from build123d import *

# Parameters (mm, degrees)
F0_R         = 16.5
F0_R_2       = 3.5170103203
F1_DEPTH     = 40
F2_R         = 16.5
F3_DEPTH     = 38
F4_W         = 50
F4_H         = 34
F5_DEPTH     = 4.5
F6_W         = 50
F6_H         = 2.5
F7_DEPTH     = 4.5
F8_T1_DEPTH  = 1.5
F8_T3_DEPTH  = 24
F8_T5_DEPTH  = 32.3129968036
F8_T7_DEPTH  = 12.8102496977
F8_T9_DEPTH  = 43
F8_T11_DEPTH = 26.1042093904
F8_T13_DEPTH = 10
F8_T20_ANGLE = 69.5823366889
F8_T22_ANGLE = 20.4176633111
F8_T24_ANGLE = 90
F8_T26_ANGLE = 90
F8_T28_ANGLE = 90
F8_T30_ANGLE = 90
F8_T32_ANGLE = 90
F9_R         = 1


# Not quite as in the source:
# - a fillet or chamfer that OpenCascade refuses, or shapes differently, is made with other operations: its cross-section is extruded or revolved along the edge and cut away or added


with BuildPart() as f1:
    # F0 (on Top) → F1 (new body)
    with BuildSketch(Plane.XY):
        with BuildLine():
            Line((0, 38), (0, 0))
            Line((0, 0), (12.5, 0))
            Line((12.5, 0), (12.5, -4.5))
            Line((12.5, -4.5), (62.5, -4.5))
            Line((62.5, -4.5), (62.5, 0))
            Line((62.5, 0), (75, 0))
            Line((75, 0), (75, 21.1042093904))
            ThreePointArc((75, 21.1042093904), (71.4247434001, 32.5159491456), (61.9772195759, 39.8476991132))
            Line((61.9772195759, 39.8476991132), (31.6943034009, 51.120442806))
            ThreePointArc((31.6943034009, 51.120442806), (29.2915599077, 51.7783562025), (26.8102496977, 52))
            Line((26.8102496977, 52), (14, 52))
            ThreePointArc((14, 52), (4.1005050634, 47.8994949366), (0, 38))
        make_face()
        with Locations((54.5, 20.5)):
            Circle(F0_R, mode=Mode.SUBTRACT)
        with BuildLine():
            ThreePointArc((4, 38), (6.9289321881, 45.0710678119), (14, 48))
            Line((14, 48), (24, 48))
            ThreePointArc((24, 48), (31.0710678119, 45.0710678119), (34, 38))
            Line((34, 38), (34, 14))
            ThreePointArc((34, 14), (31.0710678119, 6.9289321881), (24, 4))
            Line((24, 4), (14, 4))
            ThreePointArc((14, 4), (6.9289321881, 6.9289321881), (4, 14))
            Line((4, 14), (4, 38))
        make_face(mode=Mode.SUBTRACT)
        with Locations((41.3257834749, 40.5812550323)):
            Circle(F0_R_2, mode=Mode.SUBTRACT)
        with Locations((54.5, 20.5)):
            Circle(F0_R)
    extrude(amount=F1_DEPTH)

    # F2 (on face) → F3 (cut)
    with BuildSketch(Plane.XY.offset(40)):
        with Locations((54.5, 20.5)):
            Circle(F2_R)
    extrude(amount=-F3_DEPTH, mode=Mode.SUBTRACT)

    # F4 (on face) → F5 (cut)
    with BuildSketch(Plane.XZ.offset(4.5)):
        with Locations((37.5, 17)):
            Rectangle(F4_W, F4_H)
    extrude(amount=-F5_DEPTH, mode=Mode.SUBTRACT)

    # F6 (on face) → F7 (cut)
    with BuildSketch(Plane(origin=(0, 0, 34), x_dir=(1, 0, 0), z_dir=(0, 0, -1))):
        with Locations((37.5, 1.25)):
            Rectangle(F6_W, F6_H)
    extrude(amount=-F7_DEPTH, mode=Mode.SUBTRACT)

    # F8: fillet of radius 2 on 6 edges, made by hand

    # F8_s2 → F8_t1 (join)
    with BuildSketch(Plane.XY.offset(38.5)):
        with BuildLine():
            ThreePointArc((10.5, 0), (11.9142135624, -0.5857864376), (12.5, -2))
            Line((12.5, -2), (12.5, 0))
            Line((12.5, 0), (10.5, 0))
        make_face()
        with BuildLine():
            ThreePointArc((64.5, 0), (63.0857864376, -0.5857864376), (62.5, -2))
            Line((62.5, -2), (62.5, 0))
            Line((62.5, 0), (64.5, 0))
        make_face()
    extrude(amount=F8_T1_DEPTH)

    # F8_s4 → F8_t3 (cut)
    with BuildSketch(Plane.XZ.offset(-38)):
        with BuildLine():
            ThreePointArc((36, 40), (34.5857864376, 39.4142135624), (34, 38))
            Line((34, 38), (34, 40))
            Line((34, 40), (36, 40))
        make_face()
        with BuildLine():
            ThreePointArc((2, 40), (3.4142135624, 39.4142135624), (4, 38))
            Line((4, 38), (4, 40))
            Line((4, 40), (2, 40))
        make_face()
    extrude(amount=F8_T3_DEPTH, mode=Mode.SUBTRACT)

    # F8_s6 → F8_t5 (cut)
    with BuildSketch(Plane(origin=(41.4063945876, -15.4134321387, 0), x_dir=(0, 0, 1), z_dir=(-0.9371744861, 0.3488609788, 0))):
        with BuildLine():
            ThreePointArc((40, 56.9656804247), (39.4142135624, 58.3798939871), (38, 58.9656804247))
            Line((38, 58.9656804247), (40, 58.9656804247))
            Line((40, 58.9656804247), (40, 56.9656804247))
        make_face()
    extrude(amount=F8_T5_DEPTH, mode=Mode.SUBTRACT)

    # F8_s8 → F8_t7 (cut)
    with BuildSketch(Plane.YZ.offset(14)):
        with BuildLine():
            ThreePointArc((50, 40), (51.4142135624, 39.4142135624), (52, 38))
            Line((52, 38), (52, 40))
            Line((52, 40), (50, 40))
        make_face()
    extrude(amount=F8_T7_DEPTH, mode=Mode.SUBTRACT)

    # F8_s10 → F8_t9 (cut)
    with BuildSketch(Plane.XZ.offset(-38)):
        with BuildLine():
            ThreePointArc((2, 40), (0.5857864376, 39.4142135624), (0, 38))
            Line((0, 38), (0, 40))
            Line((0, 40), (2, 40))
        make_face()
    extrude(amount=F8_T9_DEPTH, mode=Mode.SUBTRACT)

    # F8_s12 → F8_t11 (cut)
    with BuildSketch(Plane.XZ.offset(-21.1042093904)):
        with BuildLine():
            ThreePointArc((73, 40), (74.4142135624, 39.4142135624), (75, 38))
            Line((75, 38), (75, 40))
            Line((75, 40), (73, 40))
        make_face()
    extrude(amount=F8_T11_DEPTH, mode=Mode.SUBTRACT)

    # F8_s14 → F8_t13 (cut)
    with BuildSketch(Plane.YZ.offset(14)):
        with BuildLine():
            ThreePointArc((2, 40), (3.4142135624, 39.4142135624), (4, 38))
            Line((4, 38), (4, 40))
            Line((4, 40), (2, 40))
        make_face()
        with BuildLine():
            ThreePointArc((50, 40), (48.5857864376, 39.4142135624), (48, 38))
            Line((48, 38), (48, 40))
            Line((48, 40), (50, 40))
        make_face()
    extrude(amount=F8_T13_DEPTH, mode=Mode.SUBTRACT)

    # F8_s15 → F8_t16 (revolve, cut)
    with BuildSketch(Plane.XZ.offset(-20.5)):
        with BuildLine():
            ThreePointArc((73, 40), (71.5857864376, 39.4142135624), (71, 38))
            Line((71, 38), (71, 40))
            Line((71, 40), (73, 40))
        make_face()
    revolve(axis=Axis((54.5, 20.5, 40), (0, 0, 1)), mode=Mode.SUBTRACT)

    # F8_s17 → F8_t18 (revolve, cut)
    with BuildSketch(Plane.XZ.offset(-40.5812550323)):
        with BuildLine():
            ThreePointArc((46.8427937951, 40), (45.4285802328, 39.4142135624), (44.8427937951, 38))
            Line((44.8427937951, 38), (44.8427937951, 40))
            Line((44.8427937951, 40), (46.8427937951, 40))
        make_face()
    revolve(axis=Axis((41.3257834749, 40.5812550323, 40), (0, 0, 1)), mode=Mode.SUBTRACT)

    # F8_s19 → F8_t20 (revolve, cut)
    with BuildSketch(Plane.XZ.offset(-21.1042093904)):
        with BuildLine():
            ThreePointArc((73, 40), (74.4142135624, 39.4142135624), (75, 38))
            Line((75, 38), (75, 40))
            Line((75, 40), (73, 40))
        make_face()
    revolve(axis=Axis((55, 21.1042093904, 40), (0, 0, 1)), revolution_arc=F8_T20_ANGLE, mode=Mode.SUBTRACT)

    # F8_s21 → F8_t22 (revolve, cut)
    with BuildSketch(Plane(origin=(11.1234784125, -4.140688446, 0), x_dir=(0, 0, 1), z_dir=(0.9371744861, -0.3488609788, 0))):
        with BuildLine():
            ThreePointArc((38, -58.9656804247), (39.4142135624, -58.3798939871), (40, -56.9656804247))
            Line((40, -56.9656804247), (40, -58.9656804247))
            Line((40, -58.9656804247), (38, -58.9656804247))
        make_face()
    revolve(axis=Axis((26.8102496977, 38, 40), (0, 0, 1)), revolution_arc=F8_T22_ANGLE, mode=Mode.SUBTRACT)

    # F8_s23 → F8_t24 (revolve, cut)
    with BuildSketch(Plane.YZ.offset(14)):
        with BuildLine():
            ThreePointArc((50, 40), (51.4142135624, 39.4142135624), (52, 38))
            Line((52, 38), (52, 40))
            Line((52, 40), (50, 40))
        make_face()
    revolve(axis=Axis((14, 38, 40), (0, 0, 1)), revolution_arc=F8_T24_ANGLE, mode=Mode.SUBTRACT)

    # F8_s25 → F8_t26 (revolve, cut)
    with BuildSketch(Plane.YZ.offset(24)):
        with BuildLine():
            ThreePointArc((50, 40), (48.5857864376, 39.4142135624), (48, 38))
            Line((48, 38), (48, 40))
            Line((48, 40), (50, 40))
        make_face()
    revolve(axis=Axis((24, 38, 40), (0, 0, -1)), revolution_arc=F8_T26_ANGLE, mode=Mode.SUBTRACT)

    # F8_s27 → F8_t28 (revolve, cut)
    with BuildSketch(Plane.XZ.offset(-14)):
        with BuildLine():
            ThreePointArc((36, 40), (34.5857864376, 39.4142135624), (34, 38))
            Line((34, 38), (34, 40))
            Line((34, 40), (36, 40))
        make_face()
    revolve(axis=Axis((24, 14, 40), (0, 0, -1)), revolution_arc=F8_T28_ANGLE, mode=Mode.SUBTRACT)

    # F8_s29 → F8_t30 (revolve, cut)
    with BuildSketch(Plane.YZ.offset(14)):
        with BuildLine():
            ThreePointArc((2, 40), (3.4142135624, 39.4142135624), (4, 38))
            Line((4, 38), (4, 40))
            Line((4, 40), (2, 40))
        make_face()
    revolve(axis=Axis((14, 14, 40), (0, 0, -1)), revolution_arc=F8_T30_ANGLE, mode=Mode.SUBTRACT)

    # F8_s31 → F8_t32 (revolve, cut)
    with BuildSketch(Plane.XZ.offset(-38)):
        with BuildLine():
            ThreePointArc((2, 40), (3.4142135624, 39.4142135624), (4, 38))
            Line((4, 38), (4, 40))
            Line((4, 40), (2, 40))
        make_face()
    revolve(axis=Axis((14, 38, 40), (0, 0, -1)), revolution_arc=F8_T32_ANGLE, mode=Mode.SUBTRACT)

    # F9
    f9_edges = [f1.edges().sort_by_distance(p)[0] for p in [
        (37.5, -4.5, 40),
    ]]
    fillet(f9_edges, radius=F9_R)


solid = f1.part
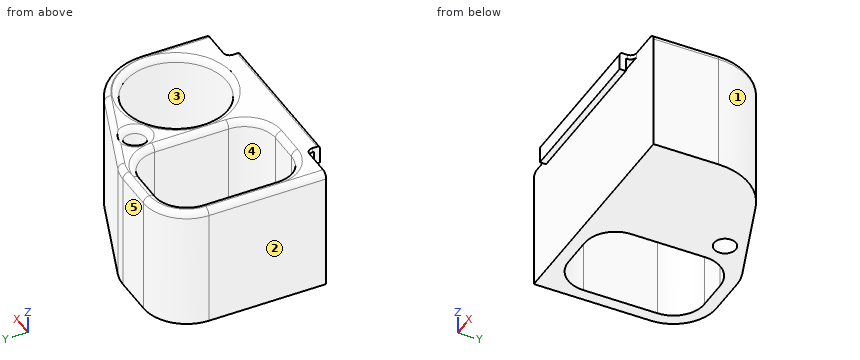
The model under review builds one solid part; all positions refer to its coordinate system, in mm. Face numbers are marked on the shaded views. A direction names the side the tool comes from. Give positions to 0.01 mm unless a question says otherwise; leave off trailing zeros. Write each loop counter-clockwise with the first axis right and the second up, starting at its lowest first coordinate (ties: lowest second). Pieces come first, ordered by that corner, then holes. Notation, with made-up numbers: M -27,-2 L 13,-2 A22 ccw 13,32 Z; hole C -10,2 d2. An arc over 180 degrees is marked long. One line per question, with ' | ' between items. Start each with the question number.
Item 1: We need section B-B on z = 36. Write out the cut boundary in (x, y).
Item 2: Draft analysis for pull direction X (two halves, no side actions). For the marked faces 1, 2 and 3, state which applies: released by +X, released by -X, zero draft, split by the parting line, or undercut.
Item 3: For the marked faces 4 and 5, list the 3-axis set-ups (+Z, -Z, +X, -X, +Y, -Y) from which the entire face can be reached by the end or side of a thin tool; tool diameter is ignored.
Item 4: Wall thickness on line 1 (X direction, y = 20, z = 20); line 2 (X direction, y = 18, z = 16); line 3 (Y direction, x = 41, z = 7.5): over which ranges is each line inside the solid? List them lowest first. Write a range as from..to.
Item 5: For pin 1 (5 mm diameter, centred on x = 27, z = 37, fed in from +Y); pin 2 (8 mm diameter, centred on x = 21.5, y = 45, fed in from +Z); pin 3 (1.5 mm diameter, centred on x = 55, y = 41.5, fed in from +Z); pin 4 (1.6 mm diameter, centred on x = 46.5, y = -4, fed in from -Z), all flat-tipped, find the tip position at first contact; note any pin that passes through.
Item 6: We need section A-A on x = 15. Write out the cut boundary in (y, z).
Item 7: We need section C-C on z = 8. Write out the cut boundary in (x, y), plus the area to 3 significant figures.
Results found:
1) outline: M 0,0 L 75,0 L 75,21.1 A20 ccw 61.98,39.85 L 31.69,51.12 A14 ccw 26.81,52 L 14,52 A14 ccw 0,38 Z; M 12.5,-4.5 L 62.5,-4.5 L 62.5,-2.5 L 12.5,-2.5 Z; hole M 4,14 A10 ccw 14,4 L 24,4 A10 ccw 34,14 L 34,38 A10 ccw 24,48 L 14,48 A10 ccw 4,38 Z; hole C 41.33,40.58 d7.03; hole C 54.5,20.5 d33
2) face 1: released by +X | face 2: released by -X | face 3: undercut
3) face 4: +Z, -Z | face 5: +Z, -Z, +X, -X, +Y
4) line 1: x = 0..4, 34..38.01, 70.99..75 | line 2: x = 0..4, 34..38.19, 70.81..75 | line 3: y = 0..11.01, 29.99..37.08, 44.08..47.66
5) pin 1: stops at y = 52 | pin 2: stops at z = 39.73 | pin 3: stops at z = 39.97 | pin 4: stops at z = 34
6) outline: M -4.5,34 L -2.5,34 L -2.5,38.5 L 0,38.5 L 0,0 L 4,0 L 4,38 A2 ccw 2,40 L -3.5,40 A1 ccw -4.5,39 Z; M 48,0 L 52,0 L 52,38 A2 ccw 48,38 Z
7) outline: M 0,0 L 75,0 L 75,21.1 A20 ccw 61.98,39.85 L 31.69,51.12 A14 ccw 26.81,52 L 14,52 A14 ccw 0,38 Z; hole M 4,14 A10 ccw 14,4 L 24,4 A10 ccw 34,14 L 34,38 A10 ccw 24,48 L 14,48 A10 ccw 4,38 Z; hole C 41.33,40.58 d7.03; hole C 54.5,20.5 d33 | area: 1,310 mm2
